```python
from build123d import *

# Parameters (mm, degrees)
SKETCH1_R                = 6
BOSS_EXTRUDE1_DEPTH      = 2
SKETCH2_R                = 1.25
CUT_EXTRUDE1_DEPTH       = 3
CUT_EXTRUDE1_DEPTH_BACK  = 4
SKETCH3_R                = 2
SKETCH3_R_2              = 0.75
BOSS_EXTRUDE2_DEPTH      = 0.2
BOSS_EXTRUDE2_DEPTH_BACK = 2.2
BOSS_EXTRUDE3_DEPTH      = 2
CIRPATTERN1_COUNT        = 18
SKETCH5_R                = 2.5
CUT_EXTRUDE2_DEPTH       = 3
CUT_EXTRUDE2_DEPTH_BACK  = 5


with BuildPart() as part:
    # Sketch1 → Boss-Extrude1 (new body)
    with BuildSketch(Plane(origin=(0, 0, 0), x_dir=(1, 0, 0), z_dir=(0, 1, 0))):
        Circle(SKETCH1_R)
    extrude(amount=BOSS_EXTRUDE1_DEPTH)

    # Sketch2 → Cut-Extrude1 (cut, two sides)
    with BuildSketch(Plane(origin=(0, 2, 0), x_dir=(1, 0, 0), z_dir=(0, 1, 0))) as cut_extrude1_sk:
        Circle(SKETCH2_R)
    extrude(amount=CUT_EXTRUDE1_DEPTH, mode=Mode.SUBTRACT)
    extrude(cut_extrude1_sk.sketch, amount=-CUT_EXTRUDE1_DEPTH_BACK, mode=Mode.SUBTRACT)

    # Sketch3 → Boss-Extrude2 (add, two sides)
    with BuildSketch(Plane(origin=(0, 2, 0), x_dir=(1, 0, 0), z_dir=(0, 1, 0))) as boss_extrude2_sk:
        Circle(SKETCH3_R)
        Circle(SKETCH3_R_2, mode=Mode.SUBTRACT)
    extrude(amount=BOSS_EXTRUDE2_DEPTH)
    extrude(boss_extrude2_sk.sketch, amount=-BOSS_EXTRUDE2_DEPTH_BACK)

    # Sketch4 → Boss-Extrude3 (add)
    with BuildSketch(Plane(origin=(0, 2, 0), x_dir=(1, 0, 0), z_dir=(0, 1, 0))):
        with BuildLine():
            Line((-0.3, 7.3), (0.3, 7.3))
            ThreePointArc((0.3, 7.3), (0.517384179, 6.661411125), (0.65, 6))
            Line((0.65, 6), (0.65, 5.964687754))
            ThreePointArc((0.65, 5.964687754), (0, 6), (-0.65, 5.964687754))
            Line((-0.65, 5.964687754), (-0.65, 6))
            ThreePointArc((-0.65, 6), (-0.512944228, 6.660215754), (-0.3, 7.3))
        make_face()
    boss_extrude3 = extrude(amount=-BOSS_EXTRUDE3_DEPTH)

    # CirPattern1: Boss-Extrude3 ×18 about axis
    cirpattern1_axis = Axis((0, 0, 0), (0, 1, 0))
    for i in range(1, CIRPATTERN1_COUNT):
        add(boss_extrude3.rotate(cirpattern1_axis, i * 360 / CIRPATTERN1_COUNT))

    # Sketch5 → Cut-Extrude2 (cut, two sides)
    with BuildSketch(Plane(origin=(0, 2, 0), x_dir=(1, 0, 0), z_dir=(0, 1, 0))) as cut_extrude2_sk:
        Circle(SKETCH5_R)
    extrude(amount=CUT_EXTRUDE2_DEPTH, mode=Mode.SUBTRACT)
    extrude(cut_extrude2_sk.sketch, amount=-CUT_EXTRUDE2_DEPTH_BACK, mode=Mode.SUBTRACT)


solid = part.part
```
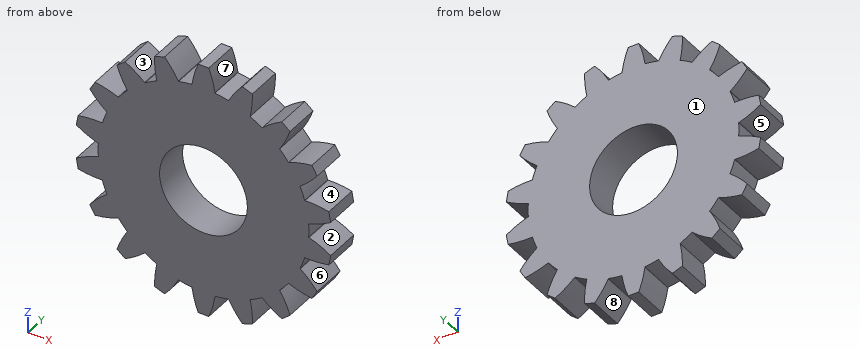
Input: part model. Units: mm. Frame: model coordinates. Face numbers are marked on the shaded views. A direction names the side the tool comes from. Round coordinates to 2 decimals unless told otherwise and drop trailing zeros. Loops run counter-clockwise (first coordinate to the right, second up) from the corner with the lowest first, then second, coordinate; pieces in that order, holes last. Notation, with made-up numbers: (2.5, 55.25) -> (12.5, 55.25) arc R18 cw to (12.5, 70.25) -> close; hole circle Ø5 at (64.5, 26.5). An arc over 180 degrees is marked (long way). Write each question's results on one line, items separated by ' | '.
1. Section B-B (x = 0). Return loops of the section in (y, z).
Geometry results:
outline: (0, -7.3) -> (2, -7.3) -> (2, -2.5) -> (0, -2.5) -> close; (0, 2.5) -> (2, 2.5) -> (2, 7.3) -> (0, 7.3) -> close
2. Ray query, line 1 (X direction, y = 1, z = 0); line 2 (Z direction, x = 0, y = 0.85); line 3 (X direction, y = 0.8, z = -6.25). Return the intervals inside material, ascending. Write a range as from..to.
Geometry results:
line 1: -6..-2.5, 2.5..6 | line 2: -7.3..-2.5, 2.5..7.3 | line 3: -2.77..-1.67, -0.61..0.61, 1.67..2.78
3. First-contact query: P1, Ø1, axis at x = -4.5, y = 1.5, coming from the +Z side; P2, Ø1, axis at y = 0.5, z = 4, coming from the +X side; P3, Ø1, axis at y = 1, z = -3.5, coming from the +X side; P4, Ø3, axis at x = 0, z = 0, coming from the +Y side. Flat tips, straight axial feed; report the tip coordinate or a pass-through.
Geometry results:
P1: z = 5.78 | P2: x = 6.41 | P3: x = 6.47 | P4: through
4. Section A-A (z = 0). Return loops of the section in (x, y), and give its area (3 significant figures).
Geometry results:
outline: (-6, 0) -> (-2.5, 0) -> (-2.5, 2) -> (-6, 2) -> close; (2.5, 0) -> (6, 0) -> (6, 2) -> (2.5, 2) -> close | area: 14.0 mm2
5. Mould query, pull axis Z, two halves, no side actions, for the marked faces 1, 2, 3 and 4. Classes: +Z half, -Z half, draft (parallel to the pull), parting line (faces both ways), or undercut.
Geometry results:
face 1: draft | face 2: undercut | face 3: +Z half | face 4: undercut
6. Set-up query: the marked faces 5, 6, 7 and 8. Return all of +Z, -Z, +X, -X, +Y, -Y with unobstructed straight access to the full face (end or side cutting, diameter ignored); none if empty.
Geometry results:
face 5: -X, +Y, -Y | face 6: +X, +Y, -Y | face 7: +Z, +Y, -Y | face 8: -Z, +Y, -Y
